from build123d import *

# Parameters (mm, degrees)
EXTRUDE_1_DEPTH     = 41
SKETCH_2_W          = 35
SKETCH_2_H          = 37
CUT_EXTRUDE_1_DEPTH = 75.498322129
SKETCH_3_R          = 4
CUT_EXTRUDE_2_DEPTH = 61.621778265


with BuildPart() as part:
    # ｽｹｯﾁ1 → ﾎﾞｽ - 押し出し1 (new body)
    with BuildSketch(Plane.XY):
        Polygon((-25, -37), (25, -37), (25, 3), (-5, 3), (-5, -7), (-15, -7), (-15, 3), (-25, 3), align=None)
    extrude(amount=EXTRUDE_1_DEPTH)

    # ｽｹｯﾁ2 → ｶｯﾄ - 押し出し1 (cut, through all)
    with BuildSketch(Plane(origin=(25, 0, 0), x_dir=(0, 0, -1), z_dir=(1, 0, 0))):
        with Locations((-20.5, -18.5)):
            Rectangle(SKETCH_2_W, SKETCH_2_H)
    extrude(amount=-CUT_EXTRUDE_1_DEPTH, mode=Mode.SUBTRACT)

    # ｽｹｯﾁ3 → ｶｯﾄ - 押し出し2 (cut, through all)
    with BuildSketch(Plane.XY.offset(41)):
        with Locations((-17.5, -27)):
            Circle(SKETCH_3_R)
        with Locations((17.5, -27)):
            Circle(SKETCH_3_R)
    extrude(amount=-CUT_EXTRUDE_2_DEPTH, mode=Mode.SUBTRACT)


solid = part.part
Source: CAD feature listing. Evaluate the final solid. Frame: model axes, mm. A direction names the side the tool comes from. Give positions to 0.01 mm unless a question says otherwise; leave off trailing zeros. Write each loop counter-clockwise with the first axis right and the second up, starting at its lowest first coordinate (ties: lowest second). Pieces come first, ordered by that corner, then holes. Notation, with made-up numbers: (27.25, -5.5) -> (79.25, -5.5) arc R19 cw to (79.25, 18.5) -> close; hole circle Ø4 at (2, -0.5). An arc over 180 degrees is marked (long way). Return JSON: item names as keys, results as strings. Group by question number.
1. Section A-A, the plane z = 18. Output: boundary loops of the cut face in (x, y), then the cut area to 3 significant figures.
2. Access query for faces 1 (the face through (-5, 0.3, 20.2)), 2 (the face through (10, 3, 20)), 3 (the face through (-20, 0, 21)). Directions: +Z, -Z, +X, -X, +Y, -Y. A direction counts if a zero-diameter tool reaches every point of the face in a straight line with its end or side. Return the directions, or none.
3. Section D-D, the plane z = 39. Output: boundary loops of the cut face in (x, y).
4. Section B-B, the plane x = -17.5. Output: boundary loops of the cut face in (y, z).
5. Pin query (flat end, axial travel): pin 1 Ø10 at (x, z) = (16.5, 29) entering from -Y; pin 2 Ø7 at (x, y) = (17.5, -27) entering from -Z; pin 3 Ø8 at (y, z) = (-1.5, 25.5) entering from -X; pin 4 Ø0.9 at (x, z) = (-12.5, 40) entering from +Y. Return the tip coordinate at first contact, or that it passes through.
6. Material intervals for line 1 (Z direction, x = 3, y = -20.5); line 2 (Y direction, x = -17.5, z = 38.75); line 3 (Y direction, x = 12, z = 31), sorted ascending. Write a range as from..to.
7. Section C-C, the plane y = -27. Output: boundary loops of the cut face in (x, z).
8. Mould query, pull axis Z, two halves, no side actions, for faces 4 (the face through (10, 0, 21)), 5 (the face through (25, 1, 23)), 6 (the face through (0, -17, 41)), 7 (the face through (0, -19, 3)). Classes: +Z half, -Z half, draft (parallel to the pull), parting line (faces both ways), or undercut.
Determined:
{
 "1": {"outline": "(-25, 0) -> (-15, 0) -> (-15, 3) -> (-25, 3) -> close; (-5, 0) -> (25, 0) -> (25, 3) -> (-5, 3) -> close", "area": "120 mm2"},
 "2": {"face 1": "+Z, -Z, +Y", "face 2": "+Z, -Z, +X, -X, +Y", "face 3": "+X, -X, -Y"},
 "3": {"outline": "(-25, -37) -> (25, -37) -> (25, 3) -> (-5, 3) -> (-5, -7) -> (-15, -7) -> (-15, 3) -> (-25, 3) -> close; hole circle Ø8 at (-17.5, -27); hole circle Ø8 at (17.5, -27)"},
 "4": {"outline": "(-37, 0) -> (-31, 0) -> (-31, 3) -> (-37, 3) -> close; (-37, 38) -> (-31, 38) -> (-31, 41) -> (-37, 41) -> close; (-23, 0) -> (3, 0) -> (3, 41) -> (-23, 41) -> (-23, 38) -> (0, 38) -> (0, 3) -> (-23, 3) -> close"},
 "5": {"pin 1": "stops at y = 0", "pin 2": "passes through", "pin 3": "stops at x = -25", "pin 4": "stops at y = -7"},
 "6": {"line 1": "z = 0..3, 38..41", "line 2": "y = -37..-31, -23..3", "line 3": "y = 0..3"},
 "7": {"outline": "(-25, 0) -> (-21.5, 0) -> (-21.5, 3) -> (-25, 3) -> close; (-25, 38) -> (-21.5, 38) -> (-21.5, 41) -> (-25, 41) -> close; (-13.5, 0) -> (13.5, 0) -> (13.5, 3) -> (-13.5, 3) -> close; (-13.5, 38) -> (13.5, 38) -> (13.5, 41) -> (-13.5, 41) -> close; (21.5, 0) -> (25, 0) -> (25, 3) -> (21.5, 3) -> close; (21.5, 38) -> (25, 38) -> (25, 41) -> (21.5, 41) -> close"},
 "8": {"face 4": "undercut", "face 5": "draft", "face 6": "+Z half", "face 7": "undercut"}
}
